Could you check a few things on this model? Use its own coordinates, in mm. Give positions to 0.01 mm unless a question says otherwise; leave off trailing zeros. Loops run counter-clockwise (first coordinate to the right, second up) from the corner with the lowest first, then second, coordinate; pieces in that order, holes last. Notation, with made-up numbers: M 4.5,-30.5 L 12.5,-30.5 A17 cw 12.5,-24.5 Z; hole C 13,-15.5 d2. An arc over 180 degrees is marked long. Answer in a Markdown table with one row per item. Add a question column.
1. Thinking about a two-plate mould opening in X: for faces 1 (the cylindrical face through (-1.318, 1.437, 4.93)), 2 (the conical face through (-1.219, 5.491, 9.875)), 3 (the flat face through (-0.1, -2.4, 10)), which applies, released by +X, released by -X, zero draft, split by the parting line, or undercut?
2. If we section it at A-A on x = 0: List the corners of the cut face in (y, z) for me, then the cut area to 3 significant figures.
3. If we section it at C-C on z = 7.5: List the corners of the cut face in (x, y) for me.
4. I need wall thicknesses on line 1 along Y through (x, z) = (0, 7); line 2 along Y through (x, z) = (1, 0.75); line 3 along Z through (x, y) = (-2.75, 5.75). Which ranges of each line are inside material? Lowest first, please. Write a range as from..to.
Autodesk Inventor part; units mm, degrees
ref_plane "YZ Plane" through (0, 0, 0) normal (1, 0, 0) x (0, 1, 0)
ref_plane "XZ Plane" through (0, 0, 0) normal (0, 1, 0) x (-1, 0, 0)
ref_plane "XY Plane" through (0, 0, 0) normal (0, 0, 1) x (1, 0, 0)
sketch "Эскиз1" plane through (0, 0, 0) normal (0, 0, 1) x (1, 0, 0)
  circle A0 centre (0, 0) radius 7.5
  dimension "d0" = 15
extrude "Выдавливание1" add sketch "Эскиз1" along normal blind 10
sketch "Эскиз2" plane through (0, 0, 10) normal (0, 0, 1) x (1, 0, 0)
  point P0 (0, 0)
hole "Отверстие1" at (0, 0, 10) direction (0, 0, -1) diameter 3.9 end through all
chamfer "Фаска1" distance 2 angle 45 1 edges at (-7.5, 0, 10)
properties part number "Упор_В2" material "По умолчанию1"
Results:
| question | item | result |
|---|---|---|
| 1 | face 1 | undercut |
| 1 | face 2 | split by the parting line |
| 1 | face 3 | zero draft |
| 2 | outline | M -7.5,0 L -1.95,0 L -1.95,10 L -5.5,10 L -7.5,8 Z; M 1.95,0 L 7.5,0 L 7.5,8 L 5.5,10 L 1.95,10 Z |
| 2 | area | 107 mm2 |
| 3 | outline | C 0,0 d15; hole C 0,0 d3.9 |
| 4 | line 1 | -7.5..-1.95, 1.95..7.5 |
| 4 | line 2 | -7.43..-1.67, 1.67..7.43 |
| 4 | line 3 | 0..9.13 |
